Read the model definition and answer for the solid it produces. Units are mm, in the model's axes. A direction names the side the tool comes from. Coordinates: 2 decimals unless noted, no trailing zeros. Write each loop counter-clockwise with the first axis right and the second up, starting at its lowest first coordinate (ties: lowest second). Pieces come first, ordered by that corner, then holes. Notation, with made-up numbers: (56.5, -2) -> (64.5, -2) arc R19 ccw to (64.5, 18) -> close; hole circle Ø8 at (62, -9.75). An arc over 180 degrees is marked (long way). Use CSV: the item, a comma, the result in double quotes.
from build123d import *

# Parameters (mm, degrees)
SKETCH_2_R      = 0.35
SKETCH_3_R      = 1.25
EXTRUDE_1_DEPTH = 5


with BuildPart() as part:
    # По траектории1: sweep along a path in Эскиз1
    with BuildLine(Plane.XY) as sweep_1_path:
        Line((0, 0), (0, 12))
        ThreePointArc((0, 12), (1.5, 13.5), (3, 12))
        Line((3, 12), (3, 0))
    # Эскиз2 → По траектории1 (sweep)
    with BuildSketch(Plane(origin=(0, 0, 0), x_dir=(1, 0, 0), z_dir=(0, 1, 0))):
        Circle(SKETCH_2_R)
    sweep(path=sweep_1_path.line)

    # Эскиз3 → Вытянуть1 (add)
    with BuildSketch(Plane.XZ.offset(-5)):
        with Locations(Location((0, 0, 0), (0, 0, 270))):
            Circle(SKETCH_3_R)
    extrude(amount=-EXTRUDE_1_DEPTH)


solid = part.part
1. A cutting plane is placed at A-A (z = 0). Give the vertices of the cut face in (x, y).
Solutions:
outline,"(-1.25, 5) -> (-0.35, 5) -> (-0.35, 0) -> (0.35, 0) -> (0.35, 5) -> (1.25, 5) -> (1.25, 10) -> (0.35, 10) -> (0.35, 12) arc R1.15 cw to (2.65, 12) -> (2.65, 0) -> (3.35, 0) -> (3.35, 12) arc R1.85 ccw to (-0.35, 12) -> (-0.35, 10) -> (-1.25, 10) -> close"
2. A cutting plane is placed at C-C (x = 1.5). Give the vertices of the cut face in (y, z), and give its area (3 significant figures).
Solutions:
outline,"circle Ø0.7 at (13.5, 0)"
area,"0.385 mm^2"
3. A cutting plane is placed at B-B (y = 10.5). Give the vertices of the cut face in (x, z), and give its area (3 significant figures).
Solutions:
outline,"circle Ø0.7 at (0, 0); circle Ø0.7 at (3, 0)"
area,"0.770 mm^2"
4. A tool of negligible diameter and unlimited length cuts with its end or side. For faces 1 (the flat face through (0, 10, -1)), 2 (the flat face through (0, 5, -1)), from which of +Z, -Z, +X, -X, +Y, -Y can it reach the whole face along a straight path? Write none if from no direction.
Solutions:
face 1,"none"
face 2,"-Y"
5. Find the intervals of material crossed by line 1 along Y through (x, z) = (-0.1, -0.5); line 2 along Z through (x, y) = (0.05, 3); line 3 along X through (y, z) = (6.25, 0.85), in increasing order.
Solutions:
line 1,"y = 5 to 10"
line 2,"z = -0.35 to 0.35"
line 3,"x = -0.92 to 0.92"
6. Each of these flat-tipped pins is pushed along its axis until it touches: pin 1 Ø1.5 at (x, y) = (2.5, 12) entering from +Z; pin 2 Ø1 at (y, z) = (12.5, 0.5) entering from +X. Where does it stop, or does it pass through?
Solutions:
pin 1,"stops at z = 0.35"
pin 2,"stops at x = 3.33"
7. A cutting plane is placed at D-D (y = 5.5). Give the vertices of the cut face in (x, z).
Solutions:
outline,"circle Ø2.5 at (0, 0); circle Ø0.7 at (3, 0)"
